Can you work these out from the drawing? Everything is in mm from the part's minimum corner. A direction names the side the tool comes from. Give positions to 0.01 mm unless a question says otherwise; leave off trailing zeros. Loops run counter-clockwise (first coordinate to the right, second up) from the corner with the lowest first, then second, coordinate; pieces in that order, holes last. Notation, with made-up numbers: (-10, 31) - (29, 31) arc R8 ccw to (29, 46) - close; hole circle Ø7 at (52.25, 43). An arc over 180 degrees is marked (long way). Answer in a Markdown table with one row per item. Add a question column.
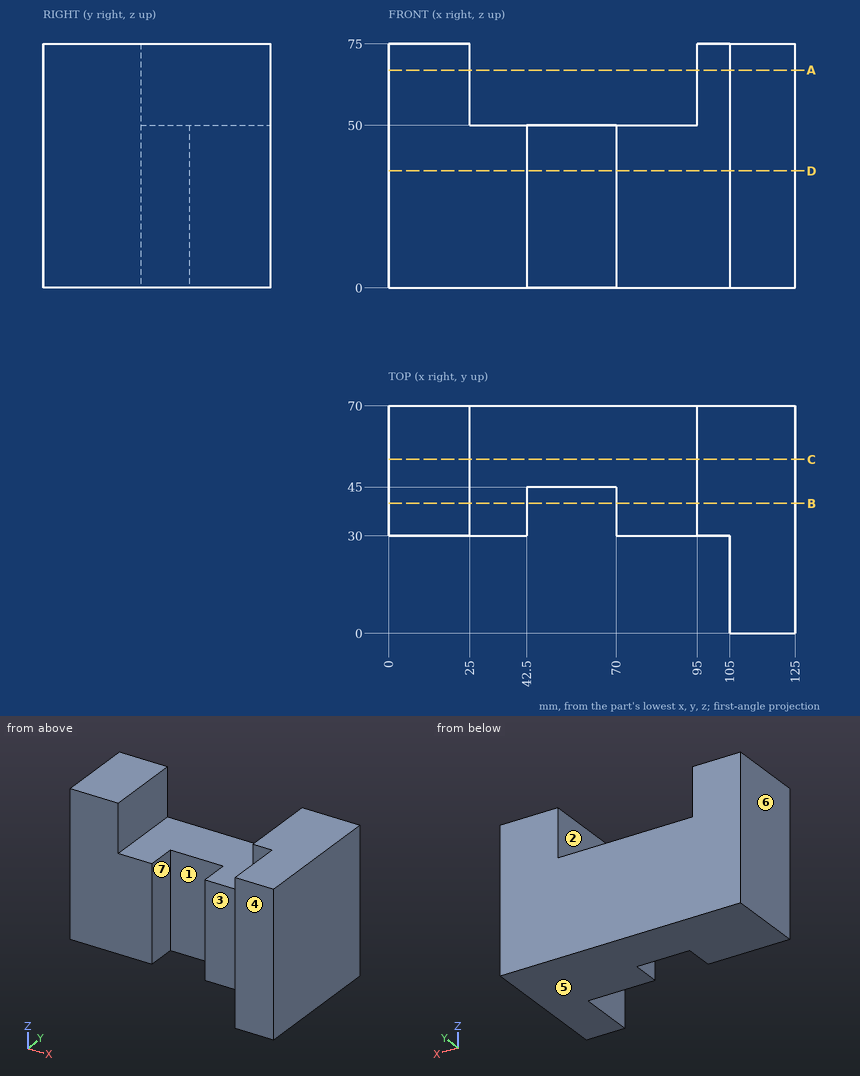
(1) For pin 1 Ø12 at (x, z) = (15.5, 40) entering from -Y; pin 2 Ø5 at (y, z) = (43.5, 28) entering from -X; pin 3 Ø14 at (x, z) = (56.5, 25.5) entering from -Y; pin 4 Ø1.5 at (x, y) = (44, 42.5) entering from -Z, each with a flat end and sliding along its axis, tell me the tip position at first contact or that it passes through.
(2) Please list where these lines run through material, in increasing order: line 1 (X direction, y = 38, z = 61); line 2 (Y direction, x = 25.5, z = 25); line 3 (Z direction, x = 50.5, y = 52).
(3) We'd pull the mould along X, two halves only. Please class the marked faces 5, 6 and 7: pulls with the +X half, pulls with the -X half, needs draft (parallel to the pull), parting line crosses it, or undercut.
(4) I want a section at D-D on z = 36. Please give me the cut outline in (x, y).
(5) I want a section at B-B on y = 40. Please give me the cut outline in (x, z).
(6) I want a section at C-C on y = 53.5. Please give me the cut outline in (x, z), then the cut area to 4 significant figures.
(7) I want a section at A-A on z = 67. Please give me the cut outline in (x, y).
(8) On a 3-axis mill with a long thin cutter (end or side, diameter ignored), from which of +Z, -Z, +X, -X, +Y, -Y can I reach the whole of each face in a straight line? I mean the marked faces 1, 2, 3 and 4. Say none if no direction works.
Reported:
| question | item | result |
|---|---|---|
| 1 | pin 1 | y = 30 |
| 1 | pin 2 | x = 0 |
| 1 | pin 3 | y = 45 |
| 1 | pin 4 | through |
| 2 | line 1 | 0 to 25, 95 to 125 |
| 2 | line 2 | 30 to 70 |
| 2 | line 3 | 0 to 50 |
| 3 | face 5 | needs draft |
| 3 | face 6 | pulls with the -X half |
| 3 | face 7 | undercut |
| 4 | outline | (0, 30) - (42.5, 30) - (42.5, 45) - (70, 45) - (70, 30) - (105, 30) - (105, 0) - (125, 0) - (125, 70) - (0, 70) - close |
| 5 | outline | (0, 0) - (42.5, 0) - (42.5, 50) - (25, 50) - (25, 75) - (0, 75) - close; (70, 0) - (125, 0) - (125, 75) - (95, 75) - (95, 50) - (70, 50) - close |
| 6 | outline | (0, 0) - (125, 0) - (125, 75) - (95, 75) - (95, 50) - (25, 50) - (25, 75) - (0, 75) - close |
| 6 | area | 7,625 mm² |
| 7 | outline | (0, 30) - (25, 30) - (25, 70) - (0, 70) - close; (95, 30) - (105, 30) - (105, 0) - (125, 0) - (125, 70) - (95, 70) - close |
| 8 | face 1 | +Z, -Z, -Y |
| 8 | face 2 | +Z, +Y, -Y |
| 8 | face 3 | +Z, -Z, -X, -Y |
| 8 | face 4 | +Z, -Z, +X, -X, -Y |
